```python
from build123d import *

# Parameters (mm, degrees)
SKETCH_1_R               = 28
EXTRUDE_1_DEPTH          = 4
SKETCH_2_R               = 12
EXTRUDE_2_DEPTH          = 22
SKETCH_3_R               = 5
CUT_EXTRUDE_1_DEPTH      = 60
SKETCH_4_R               = 1.5
CUT_EXTRUDE_2_DEPTH      = 7
PATTERN_CIRCULAR_1_COUNT = 6
SKETCH_5_R               = 1.5
CUT_EXTRUDE_3_DEPTH      = 15
SKETCH_7_R               = 7
EXTRUDE_4_DEPTH          = 10
SKETCH_8_R               = 6
CUT_EXTRUDE_4_DEPTH      = 4


with BuildPart() as part:
    # Sketch 1 → Extrude 1 (new body)
    with BuildSketch(Plane.XY):
        Circle(SKETCH_1_R)
    extrude(amount=EXTRUDE_1_DEPTH)

    # Sketch 2 → Extrude 2 (add)
    with BuildSketch(Plane.XY.offset(4)):
        Circle(SKETCH_2_R)
    extrude(amount=EXTRUDE_2_DEPTH)

    # Sketch 3 → Cut-Extrude 1 (cut)
    with BuildSketch(Plane.XY.offset(26)):
        Circle(SKETCH_3_R)
    extrude(amount=-CUT_EXTRUDE_1_DEPTH, mode=Mode.SUBTRACT)

    # Sketch 4 → Cut-Extrude 2 (cut)
    with BuildSketch(Plane(origin=(0, 0, 0), x_dir=(-1, 0, 0), z_dir=(0, 0, -1))):
        with Locations((0, 21.265645264)):
            Circle(SKETCH_4_R)
    cut_extrude_2 = extrude(amount=-CUT_EXTRUDE_2_DEPTH, mode=Mode.SUBTRACT)

    # Pattern Circular 1: Cut-Extrude 2 ×6 about axis
    pattern_circular_1_axis = Axis((0, 0, 0), (0, 0, 1))
    for i in range(1, PATTERN_CIRCULAR_1_COUNT):
        add(cut_extrude_2.rotate(pattern_circular_1_axis, i * 360 / PATTERN_CIRCULAR_1_COUNT), mode=Mode.SUBTRACT)

    # Sketch 5 → Cut-Extrude 3 (cut)
    with BuildSketch(Plane(origin=(0, 0, 0), x_dir=(1, 0, 0), z_dir=(0, 1, 0))):
        with Locations((0, -16.223306721)):
            Circle(SKETCH_5_R)
    extrude(amount=-CUT_EXTRUDE_3_DEPTH, mode=Mode.SUBTRACT)

    # Sketch 7 → Extrude 4 (add)
    with BuildSketch(Plane.XY.offset(20)):
        Circle(SKETCH_7_R)
    extrude(amount=EXTRUDE_4_DEPTH)

    # Sketch 8 → Cut-Extrude 4 (cut)
    with BuildSketch(Plane.XY.offset(30)):
        Circle(SKETCH_8_R)
    extrude(amount=-CUT_EXTRUDE_4_DEPTH, mode=Mode.SUBTRACT)


solid = part.part
```
Could you check a few things on this model? Use its own coordinates, in mm. A direction names the side the tool comes from. Coordinates: 2 decimals unless noted, no trailing zeros. Write each loop counter-clockwise with the first axis right and the second up, starting at its lowest first coordinate (ties: lowest second). Pieces come first, ordered by that corner, then holes. Notation, with made-up numbers: (27.25, 43) -> (53.25, 43) arc R20 ccw to (53.25, 69) -> close; hole circle Ø8 at (80, 88.25). An arc over 180 degrees is marked (long way). One line per question, with ' | ' between items. Start each with the question number.
1. If we section it at A-A (x = 0): Count the separate pieces of the cut face and the enclosed holes in it, and give its area (3 significant figures).
2. Please list where these lines run through material, in increasing order: line 1 along Y through (x, z) = (0, 28.2); line 2 along Y through (x, z) = (0, 1.5); line 3 along Z through (x, y) = (-1.5, -19).
3. Will these pins go through, and if not, where does the flat tip stop? P1, Ø1.5, axis at x = 8, z = 11.5, coming from the -Y side; P2, Ø3.5, axis at x = -0.5, y = 2.5, coming from the +Z side; P3, Ø6, axis at x = 11, y = -6.5, coming from the -Z side; P4, Ø12, axis at y = 0, z = 21.5, coming from the +X side.
4. For faces 4 (the face through (-0.195, -8.332, 14.736)), 5 (the face through (-13, 0, 4)), 6 (the face through (0, 0, 20)), which set-ups out of +Z, -Z, +X, -X, +Y, -Y let a thin tool reach every point of the face, with its end or its side?
5. Thinking about a two-plate mould opening in X: for faces 1 (the face through (-0.325, -19.801, 1.972)), 2 (the face through (5.2, -5.2, 26)), 3 (the face through (-11.99, 0.53, 14.85)), which applies, pulls with the +X half, pulls with the -X half, needs draft (parallel to the pull), parting line crosses it, or undercut?
6. If we section it at C-C (z = 2.5): Please give me the cut outline in (x, y).
7. If we section it at B-B (y = 20.5): Please give me the cut outline in (x, z).
8. If we section it at D-D (y = 0): Please give me the cut outline in (x, z).
Return value:
1) separate pieces: 4 | enclosed holes: 0 | area: 515 mm²
2) line 1: y = -7 to -6, 6 to 7 | line 2: y = -28 to -22.77, -19.77 to -5, 5 to 19.77, 22.77 to 28 | line 3: z = 0 to 4
3) P1: stops at y = -9.56 | P2: stops at z = 26 | P3: stops at z = 0 | P4: stops at x = 12
4) face 4: -Y | face 5: +Z | face 6: -Z
5) face 1: undercut | face 2: needs draft | face 3: parting line crosses it
6) outline: circle Ø56 at (0, 0); hole circle Ø3 at (-18.42, -10.63); hole circle Ø3 at (-18.42, 10.63); hole circle Ø10 at (0, 0); hole circle Ø3 at (0, -21.27); hole circle Ø3 at (0, 21.27); hole circle Ø3 at (18.42, -10.63); hole circle Ø3 at (18.42, 10.63)
7) outline: (-19.07, 0) -> (-1.29, 0) -> (-1.29, 4) -> (-19.07, 4) -> close; (1.29, 0) -> (19.07, 0) -> (19.07, 4) -> (1.29, 4) -> close
8) outline: (-28, 0) -> (-5, 0) -> (-5, 20) -> (5, 20) -> (5, 0) -> (28, 0) -> (28, 4) -> (12, 4) -> (12, 26) -> (7, 26) -> (7, 30) -> (6, 30) -> (6, 26) -> (-6, 26) -> (-6, 30) -> (-7, 30) -> (-7, 26) -> (-12, 26) -> (-12, 4) -> (-28, 4) -> close
